For this review, take the finished solid that the model builds, in its own axes (mm). A direction names the side the tool comes from. Give positions to 0.01 mm unless a question says otherwise; leave off trailing zeros. Order: outer loops, then holes, each group sorted by start corner. A loop starts at its lowest first (then second) coordinate and runs counter-clockwise, first axis right, second up. Notation, with made-up numbers: M -18.75,43.5 L 18.25,43.5 A7 cw 18.25,55.5 Z; hole C 8.25,46 d6. An arc over 180 degrees is marked long. Answer as CSV lines item,"result". Start each with the question number.
1. Mouldability with a two-part tool opening along X and no side actions: class faces 3 (the flat face through (-34, -30, 3.175)), 4 (the cylindrical face through (111.453, 131.872, 1.565)) as pulls with the +X half, pulls with the -X half, needs draft (parallel to the pull), parting line crosses it, or undercut.
2. Clearance check with a flat-ended pin moving along its axis: P1, Ø4.5, axis at x = -122.63, y = -32.87, coming from the -Z side. State where the tip first meets the part, or that it passes through.
3. We need section C-C, the plane z = 1.4. State how many separate pieces and enclosed holes the cut face has, and give its area (3 significant figures).
4. We need section A-A, the plane y = 111. Give the boundary of the cut face in (x, z) (3 decimals).
5. Machinability: for faces 1 (the flat face through (84.66, 96.13, 1.57)), 2 (the cylindrical face through (-94.264, -4.924, 1.565)), which of the approach directions +Z, -Z, +X, -X, +Y, -Y give a long, thin tool a straight path to every point of the face, cutting with its end or side? Answer none if there is none.
6. For line 1 along X through (y, z) = (-26, 1.05); line 2 along Y through (x, z) = (106.5, 2.1); line 3 along Y through (x, z) = (100, 0.5), list the stretches that pass through material, from the lowest coordinate up.
7. We need section B-B, the plane y = 55. Give the boundary of the cut face in (x, z) (3 decimals).
from build123d import *

# Parameters (mm, degrees)
SKETCH2_R           = 2.4892
SKETCH2_R_2         = 1.778
SKETCH2_R_3         = 10.795
SKETCH2_R_4         = 11.176
SKETCH2_R_5         = 14.2875
BOSS_EXTRUDE1_DEPTH = 3.175


with BuildPart() as part:
    # Sketch2 → Boss-Extrude1 (new body)
    with BuildSketch(Plane.XY):
        with BuildLine():
            Line((142.632381685, -29.937060043), (142.632381685, 122.462939957))
            ThreePointArc((142.632381685, 122.462939957), (134.600001748, 148.101160684), (108.918256202, 140.209048468))
            Line((108.918256202, 140.209048468), (59.7049135, 50.792022715))
            ThreePointArc((59.7049135, 50.792022715), (87.148239137, 39.915009432), (98.584532313, 12.7))
            ThreePointArc((98.584532313, 12.7), (72.574133919, -23.431032825), (30.056892785, -10.229647899))
            ThreePointArc((30.056892785, -10.229647899), (0, -31.75), (-30.056892785, -10.229647899))
            ThreePointArc((-30.056892785, -10.229647899), (-94.75382344, -3.950095664), (-59.7049135, 50.792022715))
            Line((-59.7049135, 50.792022715), (-108.918256202, 140.209048469))
            ThreePointArc((-108.918256202, 140.209048469), (-134.600001748, 148.101160684), (-142.632381685, 122.462939957))
            Line((-142.632381685, 122.462939957), (-142.632381685, -29.937060043))
            Line((-142.632381685, -29.937060043), (-142.632381685, -57.15))
            Line((-142.632381685, -57.15), (-142.632381685, -63.028571866))
            ThreePointArc((-142.632381685, -63.028571866), (-141.144484133, -66.620674314), (-137.552381685, -68.108571866))
            Line((-137.552381685, -68.108571866), (137.552381685, -68.108571866))
            ThreePointArc((137.552381685, -68.108571866), (141.144484133, -66.620674314), (142.632381685, -63.028571866))
            Line((142.632381685, -63.028571866), (142.632381685, -57.15))
            Line((142.632381685, -57.15), (142.632381685, -29.937060043))
        make_face()
        with Locations((-101.9175, -57.15)):
            Circle(SKETCH2_R, mode=Mode.SUBTRACT)
        with Locations((-89.2175, -57.15)):
            Circle(SKETCH2_R, mode=Mode.SUBTRACT)
        with Locations((-76.5175, -57.15)):
            Circle(SKETCH2_R, mode=Mode.SUBTRACT)
        with Locations((-106.68, -42.073571866)):
            Circle(SKETCH2_R_2, mode=Mode.SUBTRACT)
        with Locations((-122.627857811, -32.866071866)):
            Circle(SKETCH2_R_2, mode=Mode.SUBTRACT)
        with Locations((-122.627857811, -14.451071866)):
            Circle(SKETCH2_R_2, mode=Mode.SUBTRACT)
        with Locations((-90.732142189, -32.866071866)):
            Circle(SKETCH2_R_2, mode=Mode.SUBTRACT)
        with Locations((-106.68, -23.658571866)):
            Circle(SKETCH2_R_3, mode=Mode.SUBTRACT)
        with Locations((-90.732142189, -14.451071866)):
            Circle(SKETCH2_R_2, mode=Mode.SUBTRACT)
        with Locations((-63.8175, -57.15)):
            Circle(SKETCH2_R, mode=Mode.SUBTRACT)
        with Locations((-51.1175, -57.15)):
            Circle(SKETCH2_R, mode=Mode.SUBTRACT)
        with Locations((-38.4175, -57.15)):
            Circle(SKETCH2_R, mode=Mode.SUBTRACT)
        with Locations((-25.7175, -57.15)):
            Circle(SKETCH2_R, mode=Mode.SUBTRACT)
        with Locations((-13.0175, -57.15)):
            Circle(SKETCH2_R, mode=Mode.SUBTRACT)
        with Locations((-0.3175, -57.15)):
            Circle(SKETCH2_R, mode=Mode.SUBTRACT)
        with Locations((-106.68, -5.243571866)):
            Circle(SKETCH2_R_2, mode=Mode.SUBTRACT)
        with Locations((12.3825, -57.15)):
            Circle(SKETCH2_R, mode=Mode.SUBTRACT)
        with Locations((25.0825, -57.15)):
            Circle(SKETCH2_R, mode=Mode.SUBTRACT)
        with Locations((37.7825, -57.15)):
            Circle(SKETCH2_R, mode=Mode.SUBTRACT)
        with Locations((50.4825, -57.15)):
            Circle(SKETCH2_R, mode=Mode.SUBTRACT)
        with Locations((63.1825, -57.15)):
            Circle(SKETCH2_R, mode=Mode.SUBTRACT)
        with Locations((75.8825, -57.15)):
            Circle(SKETCH2_R, mode=Mode.SUBTRACT)
        with Locations((88.5825, -57.15)):
            Circle(SKETCH2_R, mode=Mode.SUBTRACT)
        with Locations((101.2825, -57.15)):
            Circle(SKETCH2_R, mode=Mode.SUBTRACT)
        with Locations((106.68, -42.073571866)):
            Circle(SKETCH2_R_2, mode=Mode.SUBTRACT)
        with Locations((90.732142189, -32.866071866)):
            Circle(SKETCH2_R_2, mode=Mode.SUBTRACT)
        with Locations((106.68, -23.658571866)):
            Circle(SKETCH2_R_4, mode=Mode.SUBTRACT)
        with Locations((90.732142189, -14.451071866)):
            Circle(SKETCH2_R_2, mode=Mode.SUBTRACT)
        with Locations((122.627857811, -32.866071866)):
            Circle(SKETCH2_R_2, mode=Mode.SUBTRACT)
        with Locations((122.627857811, -14.451071866)):
            Circle(SKETCH2_R_2, mode=Mode.SUBTRACT)
        with Locations((106.68, -5.243571866)):
            Circle(SKETCH2_R_2, mode=Mode.SUBTRACT)
        with Locations((-125.726814921, 131.243846084)):
            Circle(SKETCH2_R_5, mode=Mode.SUBTRACT)
        with Locations((125.726814921, 131.243846084)):
            Circle(SKETCH2_R_5, mode=Mode.SUBTRACT)
    extrude(amount=BOSS_EXTRUDE1_DEPTH)


solid = part.part
Result set:
1,face 3,"needs draft"
1,face 4,"undercut"
2,P1,"z = 0"
3,separate pieces,"1"
3,enclosed holes,"33"
3,area,"28,800 mm2"
4,outline,"M -142.632,0 L -92.842,0 L -92.842,3.175 L -142.632,3.175 Z; M 92.842,0 L 142.632,0 L 142.632,3.175 L 92.842,3.175 Z"
5,face 1,"+Z, -Z, +Y"
5,face 2,"+Z, -Z"
6,line 1,"-142.63 to -117.22, -96.14 to -18.22, 18.22 to 95.75, 117.61 to 142.63"
6,line 2,"-68.11 to -43.84, -40.3 to -34.83, -12.48 to -7.01, -3.47 to 135.82"
6,line 3,"-68.11 to -59.28, -55.02 to -32.62, -14.7 to 124.01"
7,outline,"M -142.632,0 L -62.021,0 L -62.021,3.175 L -142.632,3.175 Z; M 62.021,0 L 142.632,0 L 142.632,3.175 L 62.021,3.175 Z"
